Build history of the part. All positions in model axes, mm. Face numbers are marked on the shaded views. Round coordinates to 2 decimals unless told otherwise and drop trailing zeros. Write each loop counter-clockwise with the first axis right and the second up, starting at its lowest first coordinate (ties: lowest second). Pieces come first, ordered by that corner, then holes.
Item 1: Band-saw the part on A-A, the plane x = 0. Write the cut outline in (y, z), then the cut area to 3 significant figures.
Item 2: Mould opens along Y. For the marked faces 1 and 2 say: +Y half, -Y half, draft (parallel to the pull), parting line (faces both ways), or undercut.
Item 3: Wall check: probe 1 along Z at (x, y) = (-1.05, 1.2); probe 2 along Z at (x, y) = (-2.1, -1.8); probe 3 along X at (y, z) = (-0.15, 16.5). Give the ranges that are in metal, low to high.
Item 4: Band-saw the part on C-C, the plane z = 11. Write the cut outline in (x, y).
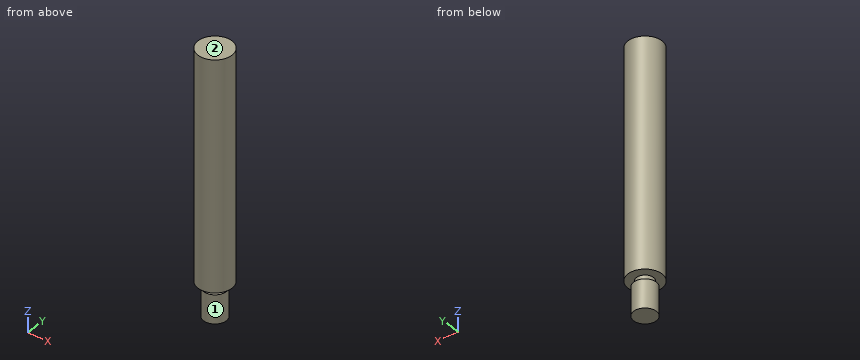
```python
from build123d import *


with BuildPart() as part:
    # Sketch1 → Revolve1 (revolve)
    with BuildSketch(Plane.XZ, mode=Mode.PRIVATE) as revolve1_sk:
        Polygon((0, 40), (3, 40), (3, 0), (1.5, 0), (1.5, -1), (2, -1), (2, -6), (0, -6), align=None)
    revolve(revolve1_sk.sketch.rotate(Axis((0, 0, 44.681241357), (0, 0, -1)), 90), axis=Axis((0, 0, 44.681241357), (0, 0, -1)))


solid = part.part
```
Results:
1. outline: (-3, 0) - (-1.5, 0) - (-1.5, -1) - (-2, -1) - (-2, -6) - (2, -6) - (2, -1) - (1.5, -1) - (1.5, 0) - (3, 0) - (3, 40) - (-3, 40) - close
1. area: 263 mm2
2. face 1: parting line
2. face 2: draft
3. probe 1: z = -6 to -1, 0 to 40
3. probe 2: z = 0 to 40
3. probe 3: x = -3 to 3
4. outline: circle Ø6 at (0, 0)
